from build123d import *

# Parameters (mm, degrees)
SKETCH1_R           = 12.5
BOSS_EXTRUDE1_DEPTH = 20
FILLET1_R           = 2.5
CUT_EXTRUDE1_REACH  = 44.205
SKETCH2_R           = 1.25
FILLET3_R           = 1
FILLET4_R           = 2.5


with BuildPart() as part:
    # Sketch1 → Boss-Extrude1 (new body)
    with BuildSketch(Plane.XY):
        with BuildLine():
            Line((-25, 6.526152156), (-15, 6.526152156))
            Line((-15, 6.526152156), (-15, 19.026152156))
            ThreePointArc((-15, 19.026152156), (0, 34.026152156), (15, 19.026152156))
            Line((15, 19.026152156), (15, 6.526152156))
            Line((15, 6.526152156), (25, 6.526152156))
            Line((25, 6.526152156), (25, 3.226152156))
            Line((25, 3.226152156), (12.5, 3.226152156))
            Line((12.5, 3.226152156), (12.5, 10.73459018))
            ThreePointArc((12.5, 10.73459018), (0, 4.026152156), (-12.5, 10.73459018))
            Line((-12.5, 10.73459018), (-12.5, 3.226152156))
            Line((-12.5, 3.226152156), (-25, 3.226152156))
            Line((-25, 3.226152156), (-25, 6.526152156))
        make_face()
        with Locations((0, 19.026152156)):
            Circle(SKETCH1_R, mode=Mode.SUBTRACT)
    extrude(amount=BOSS_EXTRUDE1_DEPTH)

    # Fillet1
    fillet1_edges = [part.edges().sort_by_distance(p)[0] for p in [
        (-15, 6.526152156, 10),
        (15, 6.526152156, 10),
    ]]
    fillet(fillet1_edges, radius=FILLET1_R)

    # Sketch2 → Cut-Extrude1 (cut, up to next)
    with BuildSketch(Plane(origin=(0, 6.526152156, 0), x_dir=(1, 0, 0), z_dir=(0, 1, 0)), mode=Mode.PRIVATE) as cut_extrude1_sk1:
        with Locations(Location((-21.25, -5, 0), (0, 0, 270))):
            Circle(SKETCH2_R)
    cut_extrude1_tool1 = extrude(cut_extrude1_sk1.sketch, amount=-CUT_EXTRUDE1_REACH, mode=Mode.PRIVATE) & part.part
    # Sketch2 → Cut-Extrude1 (cut, up to next)
    with BuildSketch(Plane(origin=(0, 6.526152156, 0), x_dir=(1, 0, 0), z_dir=(0, 1, 0)), mode=Mode.PRIVATE) as cut_extrude1_sk2:
        with Locations(Location((-21.25, -15, 0), (0, 0, 270))):
            Circle(SKETCH2_R)
    cut_extrude1_tool2 = extrude(cut_extrude1_sk2.sketch, amount=-CUT_EXTRUDE1_REACH, mode=Mode.PRIVATE) & part.part
    # Sketch2 → Cut-Extrude1 (cut, up to next)
    with BuildSketch(Plane(origin=(0, 6.526152156, 0), x_dir=(1, 0, 0), z_dir=(0, 1, 0)), mode=Mode.PRIVATE) as cut_extrude1_sk3:
        with Locations(Location((21.25, -5, 0), (0, 0, 270))):
            Circle(SKETCH2_R)
    cut_extrude1_tool3 = extrude(cut_extrude1_sk3.sketch, amount=-CUT_EXTRUDE1_REACH, mode=Mode.PRIVATE) & part.part
    # Sketch2 → Cut-Extrude1 (cut, up to next)
    with BuildSketch(Plane(origin=(0, 6.526152156, 0), x_dir=(1, 0, 0), z_dir=(0, 1, 0)), mode=Mode.PRIVATE) as cut_extrude1_sk4:
        with Locations(Location((21.25, -15, 0), (0, 0, 270))):
            Circle(SKETCH2_R)
    cut_extrude1_tool4 = extrude(cut_extrude1_sk4.sketch, amount=-CUT_EXTRUDE1_REACH, mode=Mode.PRIVATE) & part.part
    add(cut_extrude1_tool1.solids().sort_by_distance((-21.25, 6.526152, 5))[0], mode=Mode.SUBTRACT)
    add(cut_extrude1_tool2.solids().sort_by_distance((-21.25, 6.526152, 15))[0], mode=Mode.SUBTRACT)
    add(cut_extrude1_tool3.solids().sort_by_distance((21.25, 6.526152, 5))[0], mode=Mode.SUBTRACT)
    add(cut_extrude1_tool4.solids().sort_by_distance((21.25, 6.526152, 15))[0], mode=Mode.SUBTRACT)

    # Fillet3
    fillet3_edges = [part.edges().sort_by_distance(p)[0] for p in [
        (-25, 6.526152156, 10),
        (25, 6.526152156, 10),
    ]]
    fillet(fillet3_edges, radius=FILLET3_R)

    # Fillet4
    fillet4_edges = [part.edges().sort_by_distance(p)[0] for p in [
        (-12.5, 3.226152156, 10),
        (12.5, 3.226152156, 10),
    ]]
    fillet(fillet4_edges, radius=FILLET4_R)


solid = part.part
Design review of the part built by this model. Coordinates are the model's own, in mm. A direction names the side the tool comes from. Give positions to 0.01 mm unless a question says otherwise; leave off trailing zeros. Loops run counter-clockwise (first coordinate to the right, second up) from the corner with the lowest first, then second, coordinate; pieces in that order, holes last. Notation, with made-up numbers: M 36,-8.75 L 66,-8.75 A20 cw 66,27.25 Z; hole C 40.25,-5 d2. An arc over 180 degrees is marked long. Answer as a JSON object with one key per item and string values.
Item 1: We need section A-A (z = 5). State the section outline as (x, y) points.
Output values:
{"outline": "M -25,3.23 L -22.5,3.23 L -22.5,6.53 L -24,6.53 A1 ccw -25,5.53 Z; M -20,3.23 L -15,3.23 A2.5 ccw -12.5,5.73 L -12.5,10.73 A15 ccw 12.5,10.73 L 12.5,5.73 A2.5 ccw 15,3.23 L 20,3.23 L 20,6.53 L 17.5,6.53 A2.5 cw 15,9.03 L 15,19.03 A15 ccw -15,19.03 L -15,9.03 A2.5 cw -17.5,6.53 L -20,6.53 Z; M 22.5,3.23 L 25,3.23 L 25,5.53 A1 ccw 24,6.53 L 22.5,6.53 Z; hole C 0,19.03 d25"}
Item 2: We need section B-B (x = -21.25). State the section outline as (y, z) points.
Output values:
{"outline": "M 3.23,0 L 6.53,0 L 6.53,3.75 L 3.23,3.75 Z; M 3.23,6.25 L 6.53,6.25 L 6.53,13.75 L 3.23,13.75 Z; M 3.23,16.25 L 6.53,16.25 L 6.53,20 L 3.23,20 Z"}
Item 3: We need section C-C (y = 27.5). State the section outline as (x, z) points, and give its area (3 significant figures).
Output values:
{"outline": "M -12.38,0 L -9.19,0 L -9.19,20 L -12.38,20 Z; M 9.19,0 L 12.38,0 L 12.38,20 L 9.19,20 Z", "area": "128 mm2"}
Item 4: Machinability: for faces 1 (the face through (-15, 14, 10)), 2 (the face through (-13.25, 3.94, 10.14)), 3 (the face through (21, 6.526, 10)), which of the approach directions +Z, -Z, +X, -X, +Y, -Y give a long, thin tool a straight path to every point of the face, cutting with its end or side? Answer none if there is none.
Output values:
{"face 1": "+Z, -Z, -X, +Y", "face 2": "+Z, -Z, -Y", "face 3": "+Z, -Z, +X, +Y"}
Item 5: For P1, Ø3, axis at y = 14.5, z = 9.5, coming from the -X side; P2, Ø5, axis at y = 14, z = 10, coming from the +X side; P3, Ø12, axis at y = 27.5, z = 6.5, coming from the +X side, all flat-tipped, find the tip position at first contact; note any pin that passes through.
Output values:
{"P1": "stops at x = -15", "P2": "stops at x = 15", "P3": "stops at x = 14.79"}
Item 6: Wall thickness on line 1 along X through (y, z) = (10, 11.5); line 2 along X through (y, z) = (5.8, 15); line 3 along Y through (x, z) = (-5, 6.75): over which ranges is each line inside the solid? List them lowest first.
Output values:
{"line 1": "x = -15 to -12.5, -11.98 to -8.65, 8.65 to 11.98, 12.5 to 15", "line 2": "x = -24.96 to -22.5, -20 to -12.5, -7.08 to 7.08, 12.5 to 20, 22.5 to 24.96", "line 3": "y = 4.88 to 7.57, 30.48 to 33.17"}
Item 7: We need section D-D (z = 1.5). State the section outline as (x, y) points, and give its area (3 significant figures).
Output values:
{"outline": "M -25,3.23 L -15,3.23 A2.5 ccw -12.5,5.73 L -12.5,10.73 A15 ccw 12.5,10.73 L 12.5,5.73 A2.5 ccw 15,3.23 L 25,3.23 L 25,5.53 A1 ccw 24,6.53 L 17.5,6.53 A2.5 cw 15,9.03 L 15,19.03 A15 ccw -15,19.03 L -15,9.03 A2.5 cw -17.5,6.53 L -24,6.53 A1 ccw -25,5.53 Z; hole C 0,19.03 d25", "area": "332 mm2"}
Item 8: Mouldability with a two-part tool opening along Z and no side actions: class faces 4 (the face through (-22.47, 4.9, 14.73)), 5 (the face through (0, 6, 0)), 6 (the face through (13.21, 3.98, 10.14)) as pulls with the +Z half, pulls with the -Z half, needs draft (parallel to the pull), parting line crosses it, or undercut.
Output values:
{"face 4": "undercut", "face 5": "pulls with the -Z half", "face 6": "needs draft"}
